Autodesk Fusion 360 part; units mm, degrees
sketch "Sketch1" plane through (0, 0, 0) normal (1, 0, 0) x (0, 0, -1)
  line L0 (0, 0) -> (-100, 0)
  line L1 (-100, 0) -> (-100, 98)
  line L2 (-100, 98) -> (0, 98)
  line L3 (0, 98) -> (0, 0)
  dimension "d1" = 100
  dimension "d2" = 98
extrude "Extrude1" add sketch "Sketch1" against normal blind 2
extrude "Extrude2" add 1 faces at (0, 32.6667, 33.3333) along direction (1, 0, 0) blind 2
extrude "Extrude3" add 1 faces at (2, 32.6667, 33.3333) along direction (1, 0, 0) blind 1
sketch "Sketch2" plane through (3, 0, 0) normal (1, 0, 0) x (0, 0, -1)
  line L0 (-100, 98) -> (0, 98)
  line L1 (0, 98) -> (0, 0)
  line L2 (0, 0) -> (-100, 0)
  line L3 (-100, 0) -> (-100, 98)
  line L4 (-100, 98) -> (-85, 98)
  line L5 (-85, 98) -> (-85, 92.5)
  line L6 (-85, 92.5) -> (-100, 92.5)
  line L7 (-100, 92.5) -> (-100, 98)
  line L8 (-100, 98) -> (-93.5, 98)
  line L9 (-93.5, 98) -> (-93.5, 83)
  line L10 (0, 98) -> (-6.5, 98)
  line L11 (-6.5, 98) -> (-6.5, 83)
  line L12 (-6.5, 83) -> (0, 83)
  line L13 (0, 83) -> (0, 98)
  line L14 (0, 98) -> (-15, 98)
  line L15 (-15, 98) -> (-15, 92.5)
  line L16 (-15, 92.5) -> (0, 92.5)
  line L17 (0, 92.5) -> (0, 98)
  line L18 (0, 0) -> (-6.5, 0)
  line L19 (-6.5, 0) -> (-6.5, 15)
  line L20 (-6.5, 15) -> (0, 15)
  line L21 (0, 15) -> (0, 0)
  line L22 (0, 0) -> (-15, 0)
  line L23 (-15, 0) -> (-15, 5.5)
  line L24 (-15, 5.5) -> (0, 5.5)
  line L25 (0, 5.5) -> (0, 0)
  line L26 (-100, 0) -> (-85, 0)
  line L27 (-85, 0) -> (-85, 5.5)
  line L28 (-85, 5.5) -> (-100, 5.5)
  line L29 (-100, 5.5) -> (-100, 0)
  line L30 (-100, 0) -> (-94.5, 0)
  line L31 (-94.5, 0) -> (-94.5, 15)
  line L32 (-94.5, 15) -> (-100, 15)
  line L33 (-100, 15) -> (-100, 0)
  circle A0 centre (-85, 95.25) radius 1.5
  circle A1 centre (-97.25, 15) radius 1.5
  circle A2 centre (-85, 2.75) radius 1.5
  circle A3 centre (-15, 2.75) radius 1.5
  circle A4 centre (-3.25, 15) radius 1.5
  circle A5 centre (-3.25, 83) radius 1.5
  circle A6 centre (-15, 95.25) radius 1.5
  line L34 (-93.5, 83) -> (-100, 83)
  line L35 (-100, 83) -> (-100, 98)
  line L36 (-100, 98) -> (-93.5, 98)
  line L37 (-93.5, 98) -> (-93.5, 83)
  circle A7 centre (-96.75, 83) radius 1.5
  dimension "d53" = 15
  dimension "d54" = 5.5
  dimension "d55" = 6.5
  dimension "d57" = 6.5
  dimension "d58" = 15
  dimension "d59" = 15
  dimension "d60" = 5.5
  dimension "d61" = 6.5
  dimension "d62" = 15
  dimension "d63" = 5.5
  dimension "d64" = 15
  dimension "d65" = 5.5
  dimension "d66" = 15
  dimension "d67" = 100
  dimension "d68" = 98
  dimension "d69" = 5.5
  dimension "d70" = 15
  dimension "d71" = 3
  dimension "d73" = 3
  dimension "d74" = 3
  dimension "d75" = 3
  dimension "d76" = 3
  dimension "d77" = 3
  dimension "d78" = 3
  dimension "d81" = 15
  dimension "d83" = 3
extrude "Extrude9" cut sketch "Sketch2" against normal blind 20 contours L5 A0 | L5 A0 | L34 A7 | L34 A7 | L15 A6 | L15 A6 | L32 A1 | L32 A1 | L12 A5 | L12 A5 | L27 A2 | L27 A2 | L20 A4 | L20 A4 | L23 A3 | L23 A3
extrude "Extrude10" cut sketch "Sketch2" against normal blind 3 contours L0 L3 L4 L6 L7 L8 L9 L35 L36 L37 | L0 L4 L5 L6 L9 A0 L37 | L3 L6 L9 L34 L35 L37 A7 | L0 L1 L2 L3 L5 L6 L9 L11 L12 L15 L16 L19 L20 L23 L24 L27 L28 L31 L32 A0 A1 A2 A3 A4 A5 A6 L34 L37 A7 | L0 L11 L14 L15 L16 A6 | L3 L28 L31 L32 L33 A1 | L0 L1 L10 L11 L13 L14 L16 L17 | L2 L3 L26 L28 L29 L30 L31 L33 | L1 L11 L12 L13 L16 A5 | L2 L26 L27 L28 L31 A2 | L1 L19 L20 L21 L24 A4 | L2 L19 L22 L23 L24 A3 | L1 L2 L18 L19 L21 L22 L24 L25
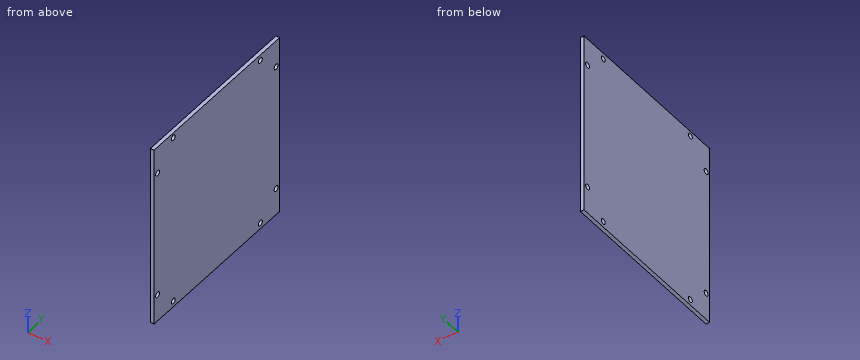
Here's how the part is built. I have some questions about the finished solid (model axes, mm). Give positions to 0.01 mm unless a question says otherwise; leave off trailing zeros. Order: outer loops, then holes, each group sorted by start corner. A loop starts at its lowest first (then second) coordinate and runs counter-clockwise, first axis right, second up. Notation, with made-up numbers: (-14.5, 13.25) -> (5.5, 13.25) arc R10 cw to (5.5, 21.25) -> close; hole circle Ø11 at (-18, 0). An arc over 180 degrees is marked (long way). Use CSV: the item, a comma, the result in double quotes. Start each with the question number.
Item 1: If I drill on probe 1 along Z at (x, y) = (-1.25, 83); probe 2 along Y at (x, z) = (-1.4, 15); probe 3 along Z at (x, y) = (-0.65, 95.25), over which ranges is the centre line in solid material (lowest first)? Write a range as [from, to].
Item 2: Suppose I cut it at A-A (z = 85). List the corners of the cut face in (x, y) for me.
Item 3: Suppose I cut it at B-B (y = 15). List the corners of the cut face in (x, z) for me, and give its area (3 significant figures).
Answer block:
1,probe 1,"z = [0, 1.75], [4.75, 95.25], [98.25, 100]"
1,probe 2,"y = [0, 1.25], [4.25, 93.75], [96.75, 98]"
1,probe 3,"z = [0, 13.5], [16.5, 83.5], [86.5, 100]"
2,outline,"(-2, 0) -> (0, 0) -> (0, 1.25) -> (-2, 1.25) -> close; (-2, 4.25) -> (0, 4.25) -> (0, 93.75) -> (-2, 93.75) -> close; (-2, 96.75) -> (0, 96.75) -> (0, 98) -> (-2, 98) -> close"
3,outline,"(-2, 0) -> (0, 0) -> (0, 1.75) -> (-2, 1.75) -> close; (-2, 4.75) -> (0, 4.75) -> (0, 95.75) -> (-2, 95.75) -> close; (-2, 98.75) -> (0, 98.75) -> (0, 100) -> (-2, 100) -> close"
3,area,"188 mm^2"
